Design review of the part built by this model. Coordinates are the model's own, in mm. A direction names the side the tool comes from. Coordinates: 2 decimals unless noted, no trailing zeros. Order: outer loops, then holes, each group sorted by start corner. A loop starts at its lowest first (then second) coordinate and runs counter-clockwise, first axis right, second up. Notation, with made-up numbers: M 38.5,-24.75 L 82.5,-24.75 A17 cw 82.5,-7.75 Z; hole C 18.25,59.25 d4. An arc over 180 degrees is marked long. Answer as a JSON object with one key per item and string values.
from build123d import *

# Parameters (mm, degrees)
SKETCH1_W                 = 30
SKETCH1_H                 = 12
BOSS_EXTRUDE1_DEPTH       = 40
SKETCH2_R                 = 5.25
CUT_EXTRUDE1_DEPTH        = 45.373415465
F_8_32_TAPPED_HOLE1_D     = 2.54
F_8_32_TAPPED_HOLE1_DEPTH = 10
F_8_32_TAPPED_HOLE1_TIP   = 0.763092986
SKETCH10_W                = 30
SKETCH10_H                = 30
SKETCH10_R                = 5.25
BOSS_EXTRUDE2_DEPTH       = 13
F_8_32_TAPPED_HOLE2_D     = 2.54
F_8_32_TAPPED_HOLE2_DEPTH = 10.71
F_8_32_TAPPED_HOLE2_TIP   = 0.763092986


with BuildPart() as part:
    # Sketch1 → Boss-Extrude1 (new body)
    with BuildSketch(Plane.XY):
        Rectangle(SKETCH1_W, SKETCH1_H)
    extrude(amount=BOSS_EXTRUDE1_DEPTH)

    # Sketch2 → Cut-Extrude1 (cut, through all)
    with BuildSketch(Plane(origin=(0, 6, 0), x_dir=(1, 0, 0), z_dir=(0, 1, 0))):
        with Locations(Location((0, -28.3, 0), (0, 0, 270))):
            Circle(SKETCH2_R)
    extrude(amount=-CUT_EXTRUDE1_DEPTH, mode=Mode.SUBTRACT)

    # #8-32 Tapped Hole1
    with Locations(Plane(origin=(0, 0, 0), x_dir=(-1, 0, 0), z_dir=(0, 0, -1))):
        with Locations((10, 0), (-10, 0)):
            Hole(F_8_32_TAPPED_HOLE1_D / 2, depth=F_8_32_TAPPED_HOLE1_DEPTH)
            with Locations((0, 0, -(F_8_32_TAPPED_HOLE1_DEPTH + F_8_32_TAPPED_HOLE1_TIP / 2))):  # 118° drill point
                Cone(0, F_8_32_TAPPED_HOLE1_D / 2, F_8_32_TAPPED_HOLE1_TIP, mode=Mode.SUBTRACT)

    # Sketch10 → Boss-Extrude2 (add)
    with BuildSketch(Plane.XZ.offset(6)):
        with Locations((0, 25)):
            Rectangle(SKETCH10_W, SKETCH10_H)
        with Locations(Location((0, 28.3, 0), (0, 0, 90))):
            Circle(SKETCH10_R, mode=Mode.SUBTRACT)
    extrude(amount=BOSS_EXTRUDE2_DEPTH)

    # #8-32 Tapped Hole2
    with Locations(Plane.ZY.offset(15)):
        with Locations((28.3, 0), (28.3, -12)):
            Hole(F_8_32_TAPPED_HOLE2_D / 2, depth=F_8_32_TAPPED_HOLE2_DEPTH)
            with Locations((0, 0, -(F_8_32_TAPPED_HOLE2_DEPTH + F_8_32_TAPPED_HOLE2_TIP / 2))):  # 118° drill point
                Cone(0, F_8_32_TAPPED_HOLE2_D / 2, F_8_32_TAPPED_HOLE2_TIP, mode=Mode.SUBTRACT)


solid = part.part
1) Add section D-D (y = -6.5). State the section outline as (x, z) points, and give its area (3 significant figures).
Taken from the geometry:
{"outline": "M -15,10 L 15,10 L 15,40 L -15,40 Z; hole C 0,28.3 d10.5", "area": "813 mm2"}
2) Add section C-C (z = 32.5). State the section outline as (x, y) points.
Taken from the geometry:
{"outline": "M -15,-19 L -3.15,-19 L -3.15,6 L -15,6 Z; M 3.15,-19 L 15,-19 L 15,6 L 3.15,6 Z"}
3) Mouldability with a two-part tool opening along X and no side actions: class faces 5 (the flat face through (0, 6, 20)), 6 (the cylindrical face through (-8.83, -0.49, 5.07)), 7 (the flat face through (-15, -6, 20)), 8 (the conical face through (-10.21, 0.07, 10.63)) as released by +X, released by -X, zero draft, split by the parting line, or undercut.
Taken from the geometry:
{"face 5": "zero draft", "face 6": "undercut", "face 7": "released by -X", "face 8": "undercut"}
4) Tool access review of faces 1 (the cylindrical face through (11.17, -0.49, 5.07)), 2 (the cylindrical face through (-9.98, 0.06, 29.57)), 3 (the flat face through (0, -6, 40)), 4 (the flat face through (0, -6, 5)): name each direction out of +Z, -Z, +X, -X, +Y, -Y from which nothing blocks a thin tool from reaching the whole face with its end or side.
Taken from the geometry:
{"face 1": "-Z", "face 2": "-X", "face 3": "+Z, +X, -X, +Y, -Y", "face 4": "-Z, +X, -X, -Y"}
5) Add section B-B (x = 0). State the section outline as (y, z) points, and give its area (4 significant figures).
Taken from the geometry:
{"outline": "M -19,10 L -6,10 L -6,0 L 6,0 L 6,23.05 L -19,23.05 Z; M -19,33.55 L 6,33.55 L 6,40 L -19,40 Z", "area": "607.5 mm2"}
6) Insertion check: pin 1 Ø4 at (x, y) = (7, -15) entering from -Z; pin 2 Ø5 at (x, z) = (5, 4) entering from -Y. Each pin has a flat end and moves straight along its axis. Give the tip position at first contact, or say it passes through.
Taken from the geometry:
{"pin 1": "stops at z = 10", "pin 2": "stops at y = -6"}
7) Add section A-A (z = 28.3). State the section outline as (x, y) points.
Taken from the geometry:
{"outline": "M -15,-19 L -5.25,-19 L -5.25,-13.27 L -15,-13.27 Z; M -15,-10.73 L -5.25,-10.73 L -5.25,-1.27 L -15,-1.27 Z; M -15,1.27 L -5.25,1.27 L -5.25,6 L -15,6 Z; M 5.25,-19 L 15,-19 L 15,6 L 5.25,6 Z"}
8) To check wall thickness, follow L1, parallel to X at y = 0, z = 6.75; L2, parallel to X at y = -9.25, z = 28.3; L3, parallel to Z at x = -11.5, y = -12. State the ranges of each line that lie inside material, in increasing order.
Taken from the geometry:
{"L1": "x = -15 to -11.27, -8.73 to 8.73, 11.27 to 15", "L2": "x = -15 to -5.25, 5.25 to 15", "L3": "z = 10 to 27.03, 29.57 to 40"}
